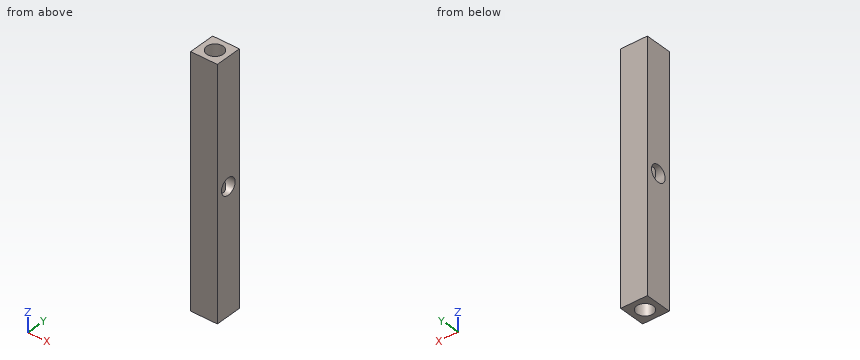
from build123d import *

# Parameters (mm, degrees)
ESBO_O1_W                  = 4.5
ESBO_O1_H                  = 41.75
RESSALTO_EXTRUS_O1_DEPTH   = 2.25
ESBO_O2_R                  = 1.4
CORTE_EXTRUS_O1_DEPTH      = 1
CORTE_EXTRUS_O1_DEPTH_BACK = 42.75
ESBO_O3_R                  = 1.4
CORTE_EXTRUS_O2_DEPTH      = 1
CORTE_EXTRUS_O2_DEPTH_BACK = 5.5


with BuildPart() as part:
    # Esboço1 → Ressalto-extrusão1 (new body, symmetric)
    with BuildSketch(Plane(origin=(0, 0, 0), x_dir=(1, 0, 0), z_dir=(0, 1, 0))):
        Rectangle(ESBO_O1_W, ESBO_O1_H)
    extrude(amount=RESSALTO_EXTRUS_O1_DEPTH, both=True)

    # Esboço2 → Corte-extrusão1 (cut, two sides)
    with BuildSketch(Plane.XY.offset(20.875)) as corte_extrus_o1_sk:
        Circle(ESBO_O2_R)
    extrude(amount=CORTE_EXTRUS_O1_DEPTH, mode=Mode.SUBTRACT)
    extrude(corte_extrus_o1_sk.sketch, amount=-CORTE_EXTRUS_O1_DEPTH_BACK, mode=Mode.SUBTRACT)

    # Esboço3 → Corte-extrusão2 (cut, two sides)
    with BuildSketch(Plane(origin=(-2.25, 0, 0), x_dir=(0, -1, 0), z_dir=(-1, 0, 0))) as corte_extrus_o2_sk:
        Circle(ESBO_O3_R)
    extrude(amount=CORTE_EXTRUS_O2_DEPTH, mode=Mode.SUBTRACT)
    extrude(corte_extrus_o2_sk.sketch, amount=-CORTE_EXTRUS_O2_DEPTH_BACK, mode=Mode.SUBTRACT)


solid = part.part
Can you work these out from the model? Positions are in its coordinate system, mm. Coordinates: 2 decimals unless noted, no trailing zeros. Loops run counter-clockwise (first coordinate to the right, second up) from the corner with the lowest first, then second, coordinate; pieces in that order, holes last. Notation, with made-up numbers: M 83,89.25 L 117,89.25 A23 ccw 117,125.25 Z; hole C 16,24 d2. An arc over 180 degrees is marked long. Return JSON: item names as keys, results as strings. Group by question number.
Item 1: Imagine slicing it at A-A (x = -0.5). Please give me the cut outline in (y, z) (3 decimals), and give its area (3 significant figures).
Item 2: If I drill on L1, parallel to X at y = 0, z = -10.5; L2, parallel to Z at x = -1.7, y = 0.15 (3 decimals), over which ranges is the centre line in solid material (lowest first)? Write a range as from..to.
Item 3: I'm going to push a flat-ended pin straight in: pin 1 Ø1.7 at (y, z) = (0, 0) entering from -X. Where does the tip first touch, or does it pass through?
Item 4: Imagine slicing it at C-C (z = 10). Please give me the cut outline in (x, y), and give its area (3 significant figures).
Item 5: Imagine slicing it at B-B (y = 0). Please give me the cut outline in (x, z) (3 decimals), and give its area (3 significant figures).
Verdict:
{
 "1": {"outline": "M -2.25,-20.875 L -1.308,-20.875 L -1.308,-0.5 A1.4 cw -1.308,0.5 L -1.308,20.875 L -2.25,20.875 Z; M 1.308,-20.875 L 2.25,-20.875 L 2.25,20.875 L 1.308,20.875 L 1.308,0.5 A1.4 cw 1.308,-0.5 Z", "area": "78.6 mm^2"},
 "2": {"L1": "x = -2.25..-1.4, 1.4..2.25", "L2": "z = -20.875..-1.392, 1.392..20.875"},
 "3": {"pin 1": "passes through"},
 "4": {"outline": "M -2.25,-2.25 L 2.25,-2.25 L 2.25,2.25 L -2.25,2.25 Z; hole C 0,0 d2.8", "area": "14.1 mm^2"},
 "5": {"outline": "M -2.25,-20.875 L -1.4,-20.875 L -1.4,-1.4 L -2.25,-1.4 Z; M -2.25,1.4 L -1.4,1.4 L -1.4,20.875 L -2.25,20.875 Z; M 1.4,-20.875 L 2.25,-20.875 L 2.25,-1.4 L 1.4,-1.4 Z; M 1.4,1.4 L 2.25,1.4 L 2.25,20.875 L 1.4,20.875 Z", "area": "66.2 mm^2"}
}
